Autodesk Inventor part; units mm, degrees
ref_plane "YZ Plane" through (0, 0, 0) normal (1, 0, 0) x (0, 1, 0)
ref_plane "XZ Plane" through (0, 0, 0) normal (0, 1, 0) x (-1, 0, 0)
ref_plane "XY Plane" through (0, 0, 0) normal (0, 0, 1) x (1, 0, 0)
sketch "Sketch1" plane through (0, 0, 0) normal (1, 0, 0) x (0, 1, 0)
  line L0 (10.2486, 23.6574) -> (0.0886, 23.6574)
  line L1 (0.0886, 23.6574) -> (0.0886, -27.1426)
  line L2 (0.0886, -27.1426) -> (10.2486, -27.1426)
  line L3 (10.2486, -27.1426) -> (10.2486, 23.6574)
  point P0 (0, 0)
  dimension "d0" = 50.8
  dimension "d1" = 10.16
extrude "Extrusion1" add sketch "Sketch1" along normal blind 2.54
sketch "Sketch2" plane through (2.54, 0, 0) normal (1, 0, 0) x (0, 0, -1)
  line L0 (-23.6574, 0.0886) -> (27.1426, 0.0886)
  line L1 (-23.6574, 10.2486) -> (-23.6574, 0.0886)
  point P0 (0, 0)
  point P1 (-10.9574, 8.2166)
  point P2 (14.4426, 8.2166)
  dimension "d4" = 0
  dimension "d5" = 8.128
  dimension "d6" = 12.7
  dimension "d7" = 25.4
hole "Hole1" at (2.54, 8.2166, 10.9574) at (2.54, 8.2166, -14.4426) direction (-1, 0, 0) diameter 3.048 end through all
properties part number "NeoPixel 8 Stick"
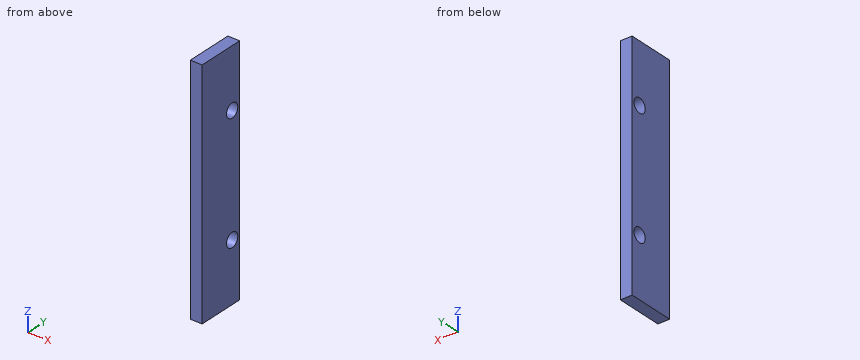
Part model, mm, in its own coordinate system. Coordinates: 2 decimals unless noted, no trailing zeros. Loops run counter-clockwise (first coordinate to the right, second up) from the corner with the lowest first, then second, coordinate; pieces in that order, holes last. Notation, with made-up numbers: (9, 28) - (41, 28) arc R30 cw to (41, 54) - close; hole circle Ø2 at (-5, -22.5). An arc over 180 degrees is marked (long way). Write item = value, one per line. Start each with the question number.
Item 1: Cut at A-A, the plane y = 7.75. Give the cut face in (x, z).
Item 2: Cut at B-B, the plane x = 0.4. Give the cut face in (y, z), and give its area (3 significant figures).
Item 3: Wall check: L1, parallel to Z at x = 2.4, y = 9.5; L2, parallel to Z at x = 2.3, y = 7; L3, parallel to Y at x = 2.3, z = -14. Give the ranges that are in metal, low to high. Write a range as from..to.
The answers:
q1.outline = (0, -27.14) - (2.54, -27.14) - (2.54, -15.89) - (0, -15.89) - close; (0, -12.99) - (2.54, -12.99) - (2.54, 9.51) - (0, 9.51) - close; (0, 12.41) - (2.54, 12.41) - (2.54, 23.66) - (0, 23.66) - close
q2.outline = (0.09, -27.14) - (10.25, -27.14) - (10.25, 23.66) - (0.09, 23.66) - close; hole circle Ø3.05 at (8.22, -14.44); hole circle Ø3.05 at (8.22, 10.96)
q2.area = 502 mm2
q3.L1 = -27.14..-15.26, -13.62..10.14, 11.78..23.66
q3.L2 = -27.14..-15.36, -13.52..10.04, 11.88..23.66
q3.L3 = 0.09..6.76, 9.67..10.25
